Geometry check sheet. Reference: the model listing, model coordinates, mm. Face numbers are marked on the shaded views. A direction names the side the tool comes from. Round coordinates to 2 decimals unless told otherwise and drop trailing zeros. Order: outer loops, then holes, each group sorted by start corner. A loop starts at its lowest first (then second) coordinate and runs counter-clockwise, first axis right, second up. Notation, with made-up numbers: (-13, 70) - (-7, 70) arc R8 ccw to (-7, 79) - close; hole circle Ø7 at (69.25, -26.75). An arc over 180 degrees is marked (long way). Return JSON: item names as keys, results as strings. Group by question number.
Q1. Sectioned sample at B-B, the plane y = 0. Record the cut outline in (x, z).
Q2. Gauge pin test, flat ends, axial feed: pin 1 Ø9 at (x, y) = (22.5, 0) entering from -Z; pin 2 Ø4 at (x, z) = (10, 14.5) entering from -Y; pin 3 Ø6 at (y, z) = (13, 33) entering from +X. Record the tip position at first contact, or that the pin passes through.
Q3. Sectioned sample at A-A, the plane x = 0. Record the cut outline in (y, z).
Q4. Material ranges on line 1 along Y through (x, z) = (-11.5, 30); line 2 along X through (y, z) = (21.5, 33.5); line 3 along Z through (x, y) = (21, -18), recorded low to high.
Q5. Draft check along Y on the marked faces 3, 4 and 5. Enter one of: pulls with the +Y half, pulls with the -Y half, needs draft (parallel to the pull), parting line crosses it, or undercut.
Q6. Sectioned sample at D-D, the plane x = -11.25. Record the cut outline in (y, z).
Q7. Sectioned sample at C-C, the plane z = 4. Record the cut outline in (x, y), then the cut area to 3 significant figures.
Q8. Tool access check on the marked faces 1 and 2. Record the directions out of +Z, -Z, +X, -X, +Y, -Y that give a thin tool (end or side, any length) a straight path to the whole face; none if there is none.
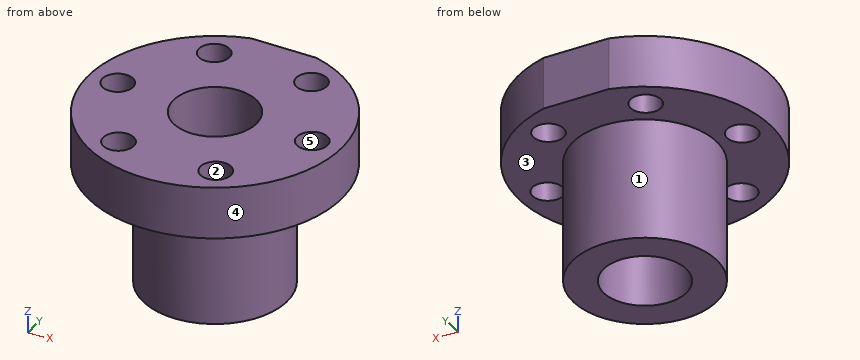
```python
from build123d import *

# Parameters (mm, degrees)
SZKIC1_R                    = 16.5
DODANIE_WYCI_GNI_CIE1_DEPTH = 28
SZKIC2_R                    = 29
DODANIE_WYCI_GNI_CIE2_DEPTH = 12
SZKIC3_R                    = 9.5
WYTNIJ_WYCI_GNI_CIE1_DEPTH  = 40
SZKIC4_W                    = 33.487046283
SZKIC4_H                    = 1
WYTNIJ_WYCI_GNI_CIE2_DEPTH  = 12
SZKIC5_R                    = 3.5
WYTNIJ_WYCI_GNI_CIE3_DEPTH  = 12
SZYK_KO_OWY1_COUNT          = 6


with BuildPart() as part:
    # Szkic1 → Dodanie-wyciągnięcie1 (new body)
    with BuildSketch(Plane.XY):
        Circle(SZKIC1_R)
    extrude(amount=DODANIE_WYCI_GNI_CIE1_DEPTH)

    # Szkic2 → Dodanie-wyciągnięcie2 (add)
    with BuildSketch(Plane.XY.offset(28)):
        Circle(SZKIC2_R)
    extrude(amount=DODANIE_WYCI_GNI_CIE2_DEPTH)

    # Szkic3 → Wytnij-wyciągnięcie1 (cut)
    with BuildSketch(Plane.XY.offset(40)):
        Circle(SZKIC3_R)
    extrude(amount=-WYTNIJ_WYCI_GNI_CIE1_DEPTH, mode=Mode.SUBTRACT)

    # Szkic4 → Wytnij-wyciągnięcie2 (cut)
    with BuildSketch(Plane.XY.offset(40)):
        with Locations((-0.738693263, 28.5)):
            Rectangle(SZKIC4_W, SZKIC4_H)
    extrude(amount=-WYTNIJ_WYCI_GNI_CIE2_DEPTH, mode=Mode.SUBTRACT)

    # Szkic5 → Wytnij-wyciągnięcie3 (cut)
    with BuildSketch(Plane.XY.offset(40)):
        with Locations((-22.5, 0)):
            Circle(SZKIC5_R)
    wytnij_wyci_gni_cie3 = extrude(amount=-WYTNIJ_WYCI_GNI_CIE3_DEPTH, mode=Mode.SUBTRACT)

    # Szyk kołowy1: Wytnij-wyciągnięcie3 ×6 about axis
    szyk_ko_owy1_axis = Axis((0, 0, 0), (0, 0, 1))
    for i in range(1, SZYK_KO_OWY1_COUNT):
        add(wytnij_wyci_gni_cie3.rotate(szyk_ko_owy1_axis, i * 360 / SZYK_KO_OWY1_COUNT), mode=Mode.SUBTRACT)


solid = part.part
```
Reply:
{
 "1": {"outline": "(-29, 28) - (-26, 28) - (-26, 40) - (-29, 40) - close; (-19, 28) - (-16.5, 28) - (-16.5, 0) - (-9.5, 0) - (-9.5, 40) - (-19, 40) - close; (9.5, 0) - (16.5, 0) - (16.5, 28) - (19, 28) - (19, 40) - (9.5, 40) - close; (26, 28) - (29, 28) - (29, 40) - (26, 40) - close"},
 "2": {"pin 1": "z = 28", "pin 2": "y = -14.43", "pin 3": "x = 27.22"},
 "3": {"outline": "(-29, 28) - (-16.5, 28) - (-16.5, 0) - (-9.5, 0) - (-9.5, 40) - (-29, 40) - close; (9.5, 0) - (16.5, 0) - (16.5, 28) - (28, 28) - (28, 40) - (9.5, 40) - close"},
 "4": {"line 1": "-26.62 to -22.98, -15.99 to 15.99, 22.98 to 26.62", "line 2": "-19.46 to -14.11, -8.39 to 8.39, 14.11 to 19.46", "line 3": "28 to 40"},
 "5": {"face 3": "needs draft", "face 4": "parting line crosses it", "face 5": "undercut"},
 "6": {"outline": "(-26.73, 28) - (-22.99, 28) - (-22.99, 40) - (-26.73, 40) - close; (-15.99, 28) - (-12.07, 28) - (-12.07, 0) - (12.07, 0) - (12.07, 28) - (15.99, 28) - (15.99, 40) - (-15.99, 40) - close; (22.99, 28) - (26.73, 28) - (26.73, 40) - (22.99, 40) - close"},
 "7": {"outline": "circle Ø33 at (0, 0); hole circle Ø19 at (0, 0)", "area": "572 mm^2"},
 "8": {"face 1": "-Z", "face 2": "+Z, -Z"}
}
